Geometry check sheet. Reference: the model listing, model coordinates, mm. Give positions to 0.01 mm unless a question says otherwise; leave off trailing zeros. Write each loop counter-clockwise with the first axis right and the second up, starting at its lowest first coordinate (ties: lowest second). Pieces come first, ordered by that corner, then holes. Notation, with made-up numbers: M 32.25,-17 L 48.25,-17 A32 ccw 48.25,17 Z; hole C 83,55.5 d2. An arc over 180 degrees is marked long. One line per item, written item: value. Start each with the question number.
1. Scan lines: line 1 (X direction, y = 0, z = 1.95); line 2 (X direction, y = 1, z = 0.95); line 3 (Y direction, x = 21, z = 2.25). Record each from-to range of solid material in increasing order.
2. Gauge pin test, flat ends, axial feed: pin 1 (3.5 mm diameter, centred on x = 19.69, y = -27.1, fed in from +Z); pin 2 (1 mm diameter, centred on y = 7, z = 2, fed in from -X); pin 3 (1 mm diameter, centred on y = 4, z = 1.5, fed in from +X). Record the tip position at first contact, or that the pin passes through.
3. Cross-section at A-A on x = 0. Record the cut outline in (y, z).
4. Release check for a two-part mould opening along X. For faces 1 (the face through (0, 0, -2)), 2 (the face through (-11, -14, 0)) record: pulls with the +X half, pulls with the -X half, needs draft (parallel to the pull), parting line crosses it, or undercut.
5. Cross-section at C-C on y = -33.5. Record the cut outline in (x, z).
6. Cross-section at D-D on z = 1.65. Count the separate pieces of the cut face and the enclosed holes in it, then the cut area to 3 significant figures.
from build123d import *

# Parameters (mm, degrees)
SKETCH1_R           = 37.5
SKETCH1_R_2         = 1.35
SKETCH1_R_3         = 2.1
BOSS_EXTRUDE1_DEPTH = 3
BOSS_EXTRUDE2_START = 2
SKETCH2_R           = 37.5
SKETCH2_R_2         = 29.5
SKETCH2_R_3         = 2.1
BOSS_EXTRUDE2_DEPTH = 2
BOSS_EXTRUDE3_START = 2
SKETCH3_R           = 11.35
SKETCH3_R_2         = 1.35
BOSS_EXTRUDE3_DEPTH = 2
FILLET2_R           = 10
FILLET3_R           = 10


with BuildPart() as part:
    # Sketch1 → Boss-Extrude1 (new body)
    with BuildSketch(Plane.XY):
        Circle(SKETCH1_R)
        with Locations((0, 8)):
            Circle(SKETCH1_R_2, mode=Mode.SUBTRACT)
        with Locations((0, -8)):
            Circle(SKETCH1_R_2, mode=Mode.SUBTRACT)
        with Locations((8, 0)):
            Circle(SKETCH1_R_2, mode=Mode.SUBTRACT)
        with Locations((-8, 0)):
            Circle(SKETCH1_R_2, mode=Mode.SUBTRACT)
        with Locations((0, 33.5)):
            Circle(SKETCH1_R_3, mode=Mode.SUBTRACT)
        with Locations((19.690805952, 27.102069312)):
            Circle(SKETCH1_R_3, mode=Mode.SUBTRACT)
        with Locations((31.860393296, 10.352069312)):
            Circle(SKETCH1_R_3, mode=Mode.SUBTRACT)
        with Locations((31.860393296, -10.352069312)):
            Circle(SKETCH1_R_3, mode=Mode.SUBTRACT)
        with Locations((19.690805952, -27.102069312)):
            Circle(SKETCH1_R_3, mode=Mode.SUBTRACT)
        with Locations((0, -33.5)):
            Circle(SKETCH1_R_3, mode=Mode.SUBTRACT)
        with Locations((-19.690805952, -27.102069312)):
            Circle(SKETCH1_R_3, mode=Mode.SUBTRACT)
        with Locations((-31.860393296, -10.352069312)):
            Circle(SKETCH1_R_3, mode=Mode.SUBTRACT)
        with Locations((-31.860393296, 10.352069312)):
            Circle(SKETCH1_R_3, mode=Mode.SUBTRACT)
        with Locations((-19.690805952, 27.102069312)):
            Circle(SKETCH1_R_3, mode=Mode.SUBTRACT)
    extrude(amount=BOSS_EXTRUDE1_DEPTH)

    # Sketch2 → Boss-Extrude2 (add)
    with BuildSketch(Plane(origin=(0, 0, 0), x_dir=(-1, 0, 0), z_dir=(0, 0, -1)).offset(BOSS_EXTRUDE2_START)):
        Circle(SKETCH2_R)
        Circle(SKETCH2_R_2, mode=Mode.SUBTRACT)
        with Locations((-19.690805952, 27.102069312)):
            Circle(SKETCH2_R_3, mode=Mode.SUBTRACT)
        with Locations((-31.860393296, 10.352069312)):
            Circle(SKETCH2_R_3, mode=Mode.SUBTRACT)
        with Locations((-31.860393296, -10.352069312)):
            Circle(SKETCH2_R_3, mode=Mode.SUBTRACT)
        with Locations((-19.690805952, -27.102069312)):
            Circle(SKETCH2_R_3, mode=Mode.SUBTRACT)
        with Locations((0, -33.5)):
            Circle(SKETCH2_R_3, mode=Mode.SUBTRACT)
        with Locations((0, 33.5)):
            Circle(SKETCH2_R_3, mode=Mode.SUBTRACT)
        with Locations((19.690805952, -27.102069312)):
            Circle(SKETCH2_R_3, mode=Mode.SUBTRACT)
        with Locations((31.860393296, -10.352069312)):
            Circle(SKETCH2_R_3, mode=Mode.SUBTRACT)
        with Locations((31.860393296, 10.352069312)):
            Circle(SKETCH2_R_3, mode=Mode.SUBTRACT)
        with Locations((19.690805952, 27.102069312)):
            Circle(SKETCH2_R_3, mode=Mode.SUBTRACT)
    extrude(amount=-BOSS_EXTRUDE2_DEPTH)

    # Sketch3 → Boss-Extrude3 (add)
    with BuildSketch(Plane(origin=(0, 0, 0), x_dir=(-1, 0, 0), z_dir=(0, 0, -1)).offset(BOSS_EXTRUDE3_START)):
        with Locations(Location((0, 0, 0), (0, 0, 180))):
            Circle(SKETCH3_R)
        with Locations((0, -8)):
            Circle(SKETCH3_R_2, mode=Mode.SUBTRACT)
        with Locations((8, 0)):
            Circle(SKETCH3_R_2, mode=Mode.SUBTRACT)
        with Locations((0, 8)):
            Circle(SKETCH3_R_2, mode=Mode.SUBTRACT)
        with Locations((-8, 0)):
            Circle(SKETCH3_R_2, mode=Mode.SUBTRACT)
    extrude(amount=-BOSS_EXTRUDE3_DEPTH)

    # Fillet2
    # the kernel refuses this fillet: 10 mm, written as the material it adds along each edge
    with BuildSketch(Plane(origin=(0, 0, 0), x_dir=(1, 0, 0), z_dir=(0, 1, 0))) as fillet2_piece_1:
        with BuildLine():
            CenterArc((17.35, 10), FILLET2_R, 233.130102354, 36.869897646)
            Line((11.35, 2), (11.23, 1.84))
            ThreePointArc((11.23, 1.84), (11.15, 1), (11.15, 0))
            Line((11.15, 0), (11.35, -0.2))
            Line((11.35, -0.2), (17.35, -0.2))
            Line((17.35, -0.2), (17.35, 0))
        make_face()
    revolve(axis=Axis((0, 0, 0), (0, 0, -1)))

    # Fillet3
    # the kernel refuses this fillet: 10 mm, written as the material it adds along each edge
    with BuildSketch(Plane(origin=(0, 0, 0), x_dir=(-1, 0, 0), z_dir=(0, -1, 0))) as fillet3_piece_1:
        with BuildLine():
            CenterArc((23.5, 10), FILLET3_R, 270, 36.869897646)
            Line((29.5, 2), (29.62, 1.84))
            ThreePointArc((29.62, 1.84), (29.7, 1), (29.7, 0))
            Line((29.7, 0), (29.5, -0.2))
            Line((29.5, -0.2), (23.5, -0.2))
            Line((23.5, -0.2), (23.5, 0))
        make_face()
    revolve(axis=Axis((0, 0, 0), (0, 0, -1)))


solid = part.part
Report:
1. line 1: x = -37.5 to -9.35, -6.65 to 6.65, 9.35 to 37.5
1. line 2: x = -37.49 to -8.91, -7.09 to 7.09, 8.91 to 37.49
1. line 3: y = -31.07 to -28.74, -25.46 to 25.46, 28.74 to 31.07
2. pin 1: passes through
2. pin 2: stops at x = -36.93
2. pin 3: stops at x = 37.34
3. outline: M -37.5,-2 L -35.6,-2 L -35.6,3 L -37.5,3 Z; M -31.4,-2 L -29.5,-2 A10 cw -23.5,0 L -17.35,0 A10 cw -11.35,-2 L -9.35,-2 L -9.35,3 L -31.4,3 Z; M -6.65,-2 L 6.65,-2 L 6.65,3 L -6.65,3 Z; M 9.35,-2 L 11.35,-2 A10 cw 17.35,0 L 23.5,0 A10 cw 29.5,-2 L 31.4,-2 L 31.4,3 L 9.35,3 Z; M 35.6,-2 L 37.5,-2 L 37.5,3 L 35.6,3 Z
4. face 1: needs draft
4. face 2: undercut
5. outline: M -16.85,-2 L -2.1,-2 L -2.1,3 L -16.85,3 Z; M 2.1,-2 L 16.85,-2 L 16.85,3 L 2.1,3 Z
6. separate pieces: 1
6. enclosed holes: 14
6. area: 4,260 mm^2
